Input: part model. Units: mm. Frame: model coordinates. Round coordinates to 2 decimals unless told otherwise and drop trailing zeros. Loops run counter-clockwise (first coordinate to the right, second up) from the corner with the lowest first, then second, coordinate; pieces in that order, holes last. Notation, with made-up numbers: (45, 63.25) -> (64, 63.25) arc R14 cw to (64, 81.25) -> close; hole circle Ø7 at (-31.5, 29). An arc over 180 degrees is marked (long way). Answer as a JSON object with one key per item and string values. Group by question number.
Item 1: Material intervals for line 1 (Y direction, x = -19.5, z = 4.15); line 2 (X direction, y = -17.5, z = 2.95); line 3 (Y direction, x = -20.5, z = 3.3), sorted ascending. Write a range as [from, to].
Item 2: Section query A-A on y = -17.4. Return loops of the section in (x, z), and give its area (3 significant figures).
Item 3: Draft query along Y for faces 1 (the flat face through (-17, 0, 3)), 2 (the cylindrical face through (-16.235, -15.913, 2.586)), 3 (the flat face through (-17, -25, 3)), 4 (the flat face through (-9.54, -12, 3)). Return one class per face: released by +Y, released by -Y, zero draft, split by the parting line, or undercut.
Item 4: Section query C-C on y = -3.8. Return loops of the section in (x, z), and give its area (3 significant figures).
Item 5: Section query B-B on z = 1.4. Return loops of the section in (x, y).
Item 6: Pin query (flat end, axial travel): pin 1 (3.5 mm diameter, centred on x = -19.59, y = -3.8, fed in from +Z). Return the tip coordinate at first contact, or that it passes through.
from build123d import *

# Parameters (mm, degrees)
F0_W     = 15.7
F0_H     = 5.1
F1_DEPTH = 25
F2_R     = 1.35
F3_DEPTH = 5.1
F4_R     = 1.5
F5_DEPTH = 5.1


with BuildPart() as f1:
    # F0 (on Front) → F1 (new body)
    with BuildSketch(Plane.XZ):
        with Locations((-17.389617, 2.55)):
            Rectangle(F0_W, F0_H)
    extrude(amount=F1_DEPTH)

    # F2 (on face) → F3 (cut)
    with BuildSketch(Plane.XY.offset(5.1)):
        with Locations((-19.589617, -3.8)):
            Circle(F2_R)
    extrude(amount=-F3_DEPTH, mode=Mode.SUBTRACT)

    # F4 (on face) → F5 (cut)
    with BuildSketch(Plane.XY.offset(5.1)):
        with Locations((-16.039617, -17.4)):
            Circle(F4_R)
    extrude(amount=-F5_DEPTH, mode=Mode.SUBTRACT)


solid = f1.part
Solved:
{
 "1": {"line 1": "[-25, -5.15], [-2.45, 0]", "line 2": "[-25.24, -17.54], [-14.54, -9.54]", "line 3": "[-25, -4.8], [-2.8, 0]"},
 "2": {"outline": "(-25.24, 0) -> (-17.54, 0) -> (-17.54, 5.1) -> (-25.24, 5.1) -> close; (-14.54, 0) -> (-9.54, 0) -> (-9.54, 5.1) -> (-14.54, 5.1) -> close", "area": "64.8 mm²"},
 "3": {"face 1": "released by +Y", "face 2": "undercut", "face 3": "released by -Y", "face 4": "zero draft"},
 "4": {"outline": "(-25.24, 0) -> (-20.94, 0) -> (-20.94, 5.1) -> (-25.24, 5.1) -> close; (-18.24, 0) -> (-9.54, 0) -> (-9.54, 5.1) -> (-18.24, 5.1) -> close", "area": "66.3 mm²"},
 "5": {"outline": "(-25.24, -25) -> (-9.54, -25) -> (-9.54, 0) -> (-25.24, 0) -> close; hole circle Ø2.7 at (-19.59, -3.8); hole circle Ø3 at (-16.04, -17.4)"},
 "6": {"pin 1": "z = 5.1"}
}
